Geometry check sheet. Reference: drawing and pictorial views, mm from the part's lowest x, y, z. A direction names the side the tool comes from. Round coordinates to 2 decimals unless told otherwise and drop trailing zeros. Order: outer loops, then holes, each group sorted by start corner. A loop starts at its lowest first (then second) coordinate and runs counter-clockwise, first axis right, second up.
Q1. Cross-section at C-C on z = 17.5. Record the cut outline in (x, y), then the cut area to 3 significant figures.
Q2. Cross-section at B-B on x = 62.5. Record the cut outline in (y, z) (1 decimal), then the cut area to 3 significant figures.
Q3. Set-up check for the marked faces 1, 2 and 3: record each of +Z, -Z, +X, -X, +Y, -Y from which the full face is reachable in a straight line by a thin tool's end or side.
Q4. Cross-section at A-A on y = 6.25. Record the cut outline in (x, z) (1 decimal).
Q5. Depth check by flat-ended pin: P1, Ø1.6, axis at x = 69.5, y = 3, coming from the +Z side; P2, Ø2, axis at y = 12, z = 6, coming from the -X side; P3, Ø8, axis at x = 12, y = 2, coming from the +Z side. Enter the tip coordinate at first touch or a pass-through.
Q6. Mould release check, pull along Z, two halves, no side actions. Record for the marked faces 4, 5 and 6: +Z half, -Z half, draft (parallel to the pull), parting line (faces both ways), or undercut.
Q7. Cross-section at D-D on x = 81.5. Record the cut outline in (y, z) (1 decimal), then the cut area to 3 significant figures.
Q8. Scan lines: probe 1 along Y at (x, z) = (64.5, 16.75); probe 2 along Z at (x, y) = (99, 4.75); probe 3 along Z at (x, y) = (94, 14.75) (1 decimal). Record each from-to range of solid material in increasing order.
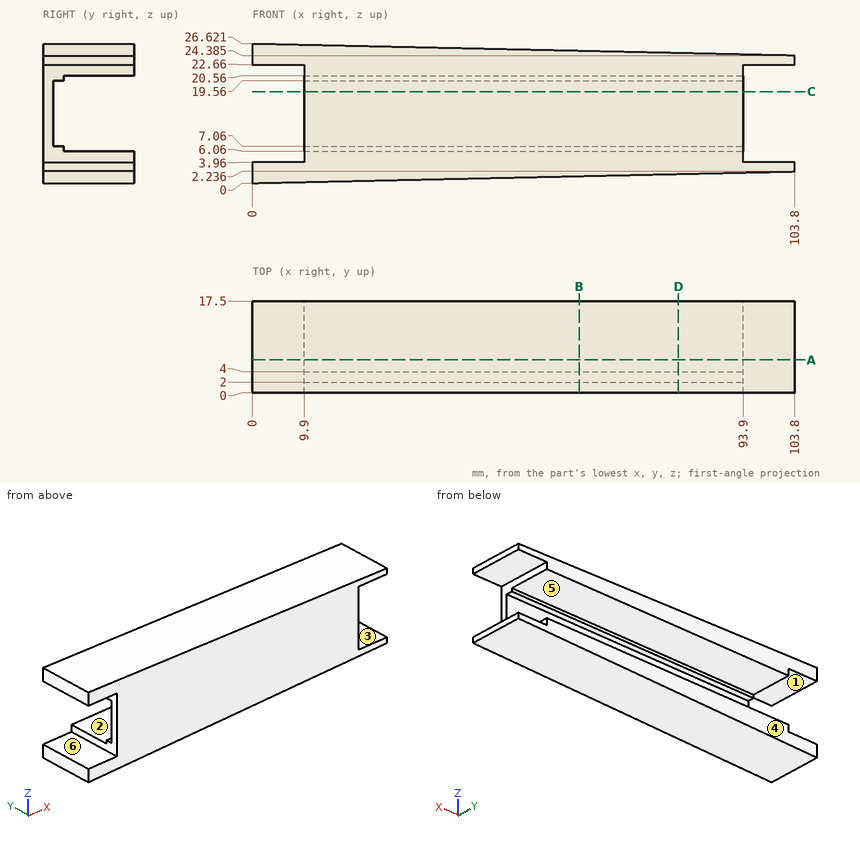
Results found:
1. outline: (9.9, 0) - (93.9, 0) - (93.9, 2) - (9.9, 2) - close
1. area: 168 mm2
2. outline: (0, 1.3) - (17.5, 1.3) - (17.5, 6.1) - (4, 6.1) - (4, 7.1) - (2, 7.1) - (2, 19.6) - (4, 19.6) - (4, 20.6) - (17.5, 20.6) - (17.5, 25.3) - (0, 25.3) - close
2. area: 198 mm2
3. face 1: -X, +Y, -Y
3. face 2: +X, -X, +Y
3. face 3: +X, +Y, -Y
4. outline: (0, 0) - (103.8, 2.2) - (103.8, 4) - (93.9, 4) - (93.9, 6.1) - (9.9, 6.1) - (9.9, 4) - (0, 4) - close; (0, 22.7) - (9.9, 22.7) - (9.9, 20.6) - (93.9, 20.6) - (93.9, 22.7) - (103.8, 22.7) - (103.8, 24.4) - (0, 26.6) - close
5. P1: stops at z = 25.14
5. P2: stops at x = 9.9
5. P3: stops at z = 26.45
6. face 4: draft
6. face 5: undercut
6. face 6: undercut
7. outline: (0, 1.8) - (17.5, 1.8) - (17.5, 6.1) - (4, 6.1) - (4, 7.1) - (2, 7.1) - (2, 19.6) - (4, 19.6) - (4, 20.6) - (17.5, 20.6) - (17.5, 24.9) - (0, 24.9) - close
7. area: 184 mm2
8. probe 1: y = 0 to 2
8. probe 2: z = 2.13 to 3.96, 22.66 to 24.49
8. probe 3: z = 2 to 4, 22.7 to 24.6
